```python
from build123d import *

# Parameters (mm, degrees)
ESQUISSE4_W              = 45
ESQUISSE4_H              = 68.965517242
BOSS_EXTRU_2_DEPTH       = 20
CONG_6_R                 = 4.310344828
ESQUISSE9_W              = 35.344827586
ESQUISSE9_H              = 58.620689655
ENL_V_MAT_EXTRU_7_DEPTH  = 14
ESQUISSE10_W             = 24.75862069
ESQUISSE10_H             = 1.613627587
ENL_V_MAT_EXTRU_8_DEPTH  = 10
ESQUISSE12_W             = 45
ESQUISSE12_H             = 68.965517242
ENL_V_MAT_EXTRU_11_DEPTH = 6.24
ESQUISSE14_W             = 6.210038645
ESQUISSE14_H             = 6.535729399
ENL_V_MAT_EXTRU_15_DEPTH = 3
ECHELLE2_SCALE           = 1.16


with BuildPart() as part:
    # Esquisse4 → Boss.-Extru.2 (new body)
    with BuildSketch(Plane.XY):
        with Locations((-111.0819834, 178.800149876)):
            Rectangle(ESQUISSE4_W, ESQUISSE4_H)
    extrude(amount=BOSS_EXTRU_2_DEPTH)

    # Congé6
    cong_6_edges = [part.edges().sort_by_distance(p)[0] for p in [
        (-133.5819834, 213.282908497, 10),
        (-88.5819834, 213.282908497, 10),
        (-88.5819834, 144.317391255, 10),
        (-133.5819834, 144.317391255, 10),
    ]]
    fillet(cong_6_edges, radius=CONG_6_R)

    # Esquisse9 → Enlèv. mat.-Extru.7 (cut)
    with BuildSketch(Plane.XY.offset(20)):
        with Locations((-111.081983607, 178.802563669)):
            Rectangle(ESQUISSE9_W, ESQUISSE9_H)
    extrude(amount=-ENL_V_MAT_EXTRU_7_DEPTH, mode=Mode.SUBTRACT)

    # Esquisse10 → Enlèv. mat.-Extru.8 (cut)
    with BuildSketch(Plane.XY.offset(20)):
        with Locations((-111.081983607, 148.685405049)):
            Rectangle(ESQUISSE10_W, ESQUISSE10_H)
    extrude(amount=-ENL_V_MAT_EXTRU_8_DEPTH, mode=Mode.SUBTRACT)

    # Esquisse12 → Enlèv. mat.-Extru.11 (cut)
    with BuildSketch(Plane.XY.offset(20)):
        with Locations((-111.0819834, 178.800149876)):
            Rectangle(ESQUISSE12_W, ESQUISSE12_H)
    extrude(amount=-ENL_V_MAT_EXTRU_11_DEPTH, mode=Mode.SUBTRACT)

    # Esquisse14 → Enlèv. mat.-Extru.15 (cut)
    with BuildSketch(Plane.XY):
        with Locations((-128.157742359, 165.722037811)):
            Rectangle(ESQUISSE14_W, ESQUISSE14_H)
        Polygon((-125.166077697, 194.70473497), (-131.262761681, 194.70473497), (-131.262761681, 175.305285642), (-124.939368374, 175.305285642), align=None)
        with BuildLine():
            add(Edge.make_bspline(
                [(-118.672815137, 173.299083951), (-119.122606069, 159.199358702), (-104.846253159, 158.743933226), (-90.56990025, 158.28850775), (-90.120109318, 172.388233)],
                knots=[0, 0, 0, 1.570796327, 1.570796327, 3.141592654, 3.141592654, 3.141592654], degree=2, weights=[1, 0.707106781, 1, 0.707106781, 1]))
            add(Edge.make_bspline(
                [(-104.31929668, 199.200388229), (-98.998777501, 190.741931467), (-90.339178369, 183.138148549), (-90.120109318, 172.388233)],
                knots=[0, 0, 0, 0, 1, 1, 1, 1], degree=3))
            add(Edge.make_bspline(
                [(-104.31929668, 199.200388229), (-109.644635947, 191.271995555), (-117.49611417, 183.324353593), (-118.672815137, 173.299083951)],
                knots=[0, 0, 0, 0, 1, 1, 1, 1], degree=3))
        make_face()
    extrude(amount=ENL_V_MAT_EXTRU_15_DEPTH, mode=Mode.SUBTRACT)


with BuildPart() as part_1:
    # Echelle2: scaled about (-111.392758629, 179.255556227, 5.432678967)
    add(part.part.scale(ECHELLE2_SCALE).moved(Location((17.822841381, -28.680888996, -0.869228635))))


solid = part_1.part
```
Can you work these out from the model? Positions are in its coordinate system, mm. A direction names the side the tool comes from. Round coordinates to 2 decimals unless told otherwise and drop trailing zeros. Order: outer loops, then holes, each group sorted by start corner. A loop starts at its lowest first (then second) coordinate and runs counter-clockwise, first axis right, second up. Notation, with made-up numbers: (-40, 89) -> (-34, 89) arc R18 ccw to (-34, 97) -> close; hole circle Ø5 at (-13.5, -5.75). An arc over 180 degrees is marked (long way). Return JSON: item names as keys, results as strings. Group by question number.
1. If we section it at D-D, the plane z = 1: Count the separate pieces of the cut face and the enclosed holes in it, then the cut area to 3 significant figures.
2. We'd pull the mould along Y, two halves only. Please class faces 4 (the face through (-111, 212.73, 11)), 5 (the face through (-135.706, 140.231, 7.223)), 6 (the face through (-135.71, 217.22, 7.22)), 7 (the face through (-131, 164, 2.611)): released by +Y, released by -Y, zero draft, split by the parting line, or undercut.
3. If we section it at C-C, the plane z = 8.75: Write out the boundary of the cut face in (x, y), then the cut area to 3 significant figures.
4. If we section it at A-A, the plane z = 12.5: Write out the boundary of the cut face in (x, y), then the cut area to 3 significant figures.
5. I need wall thicknesses on line 1 (Y direction, x = -107, z = 13.75); line 2 (X direction, y = 159.5, z = 12.75); line 3 (Z direction, x = -118.5, y = 204.5). Which ranges of each line are inside material? Lowest first, please. Write a range as [from, to].
6. Will these pins go through, and if not, where does the flat tip stop? pin 1 (20.5 mm diameter, centred on x = -103.5, y = 192, fed in from +Z); pin 2 (16.5 mm diameter, centred on x = -108, y = 172.5, fed in from -Z).
7. If we section it at B-B, the plane y = 211.5: Write out the boundary of the cut face in (x, z).
8. Which directions (+Z, -Z, +X, -X, +Y, -Y) give clear straight access to the entire face, cutting with the end or side of a thin tool? Please do faces 1 (the face through (-86.358, 217.224, 7.223)), 2 (the face through (-111, 144, 10.731)), 3 (the face through (-134.442, 186, 1)).
Output values:
{
 "1": {"separate pieces": "1", "enclosed holes": "3", "area": "2,900 mm²"},
 "2": {"face 4": "undercut", "face 5": "released by -Y", "face 6": "released by +Y", "face 7": "undercut"},
 "3": {"outline": "(-137.13, 143.73) arc R5 ccw to (-132.13, 138.73) -> (-89.93, 138.73) arc R5 ccw to (-84.93, 143.73) -> (-84.93, 213.73) arc R5 ccw to (-89.93, 218.73) -> (-132.13, 218.73) arc R5 ccw to (-137.13, 213.73) -> close; hole (-131.53, 144.73) -> (-90.53, 144.73) -> (-90.53, 212.73) -> (-131.53, 212.73) -> close", "area": "1,370 mm²"},
 "4": {"outline": "(-137.13, 143.73) arc R5 ccw to (-132.13, 138.73) -> (-89.93, 138.73) arc R5 ccw to (-84.93, 143.73) -> (-84.93, 213.73) arc R5 ccw to (-89.93, 218.73) -> (-132.13, 218.73) arc R5 ccw to (-137.13, 213.73) -> close; hole (-131.53, 144.73) -> (-125.39, 144.73) -> (-125.39, 142.86) -> (-96.67, 142.86) -> (-96.67, 144.73) -> (-90.53, 144.73) -> (-90.53, 212.73) -> (-131.53, 212.73) -> close", "area": "1,310 mm²"},
 "5": {"line 1": "[138.73, 142.86], [212.73, 218.73]", "line 2": "[-137.13, -131.53], [-90.53, -84.93]", "line 3": "[-0.87, 6.09]"},
 "6": {"pin 1": "z = 6.09", "pin 2": "z = 2.61"},
 "7": {"outline": "(-137.13, -0.87) -> (-84.93, -0.87) -> (-84.93, 15.09) -> (-90.53, 15.09) -> (-90.53, 6.09) -> (-131.53, 6.09) -> (-131.53, 15.09) -> (-137.13, 15.09) -> close"},
 "8": {"face 1": "+Z, -Z, +X, +Y", "face 2": "+Z", "face 3": "-Z"}
}
